Part model, mm, in its own coordinate system. Face numbers are marked on the shaded views. A direction names the side the tool comes from. Coordinates: 2 decimals unless noted, no trailing zeros. Write each loop counter-clockwise with the first axis right and the second up, starting at its lowest first coordinate (ties: lowest second). Pieces come first, ordered by that corner, then holes. Notation, with made-up numbers: M -28.75,-1.75 L -3.75,-1.75 A13 cw -3.75,20.25 Z; hole C -34,-27 d4. An arc over 180 degrees is marked long. Use a Markdown table: item, result. Add a question column.
Q1. Slice it at B-B on x = 14.5. Write the cut outline in (y, z).
Q2. Slice it at C-C on y = 9. Write the cut outline in (x, z).
Q3. Tool access for the marked faces 1, 2 and 3: list every direction of +Z, -Z, +X, -X, +Y, -Y with a clear straight run to the whole face (end or side of a thin tool).
Q4. Mould opens along Y. For the marked faces 4, 5, 6 and 7 say: released by +Y, released by -Y, zero draft, split by the parting line, or undercut.
Q5. Slice it at D-D on x = 3. Write the cut outline in (y, z), then the cut area to 3 significant figures.
Q6. Pin check, flat tips, straight feed: pin 1 Ø1.5 at (y, z) = (9.5, 1) entering from +X; pin 2 Ø4 at (x, y) = (-9.5, -10) entering from +Z; pin 3 Ø6.5 at (y, z) = (-4, -4) entering from +X. Stop position of each tip, or through.
Q7. Wall check: L1, parallel to Y at x = 2, z = 0.25; L2, parallel to Y at x = -5, z = 3; L3, parallel to X at y = 1, z = -2.5. Give the ranges that are in metal, low to high. Write a range as from..to.
Q8. Slice it at A-A on z = 1.25. Write the cut outline in (x, y).
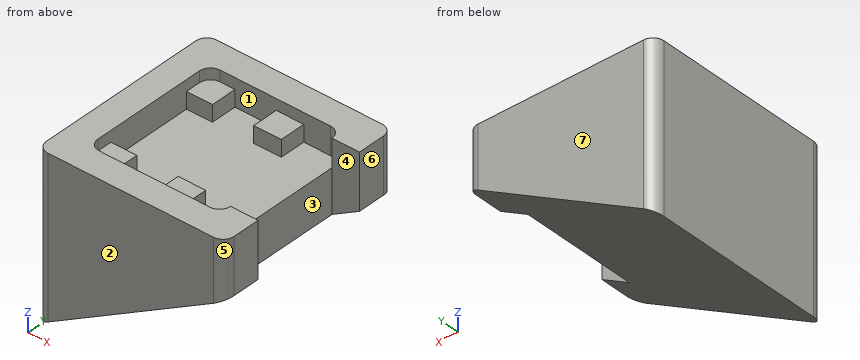
from build123d import *

# Parameters (mm, degrees)
F0_W     = 5
F0_H     = 4.7
F1_DEPTH = 5
F2_DEPTH = 3
F4_DEPTH = 2
F6_DEPTH = 35.2
F7_DEPTH = 25
F8_DEPTH = 25


with BuildPart() as f1:
    # F0 (on Top) → F1 (new body)
    with BuildSketch(Plane.XY):
        with BuildLine():
            ThreePointArc((12.031, -10.6), (11.4452135624, -12.0142135624), (10.031, -12.6))
            Line((10.031, -12.6), (5.169, -12.6))
            Line((5.169, -12.6), (0.169, -12.6))
            Line((0.169, -12.6), (-7.331, -12.6))
            Line((-7.331, -12.6), (-10.031, -12.6))
            ThreePointArc((-10.031, -12.6), (-11.4452135624, -12.0142135624), (-12.031, -10.6))
            Line((-12.031, -10.6), (-12.031, -7.9))
            Line((-12.031, -7.9), (-12.031, 7.9))
            Line((-12.031, 7.9), (-12.031, 10.6))
            ThreePointArc((-12.031, 10.6), (-11.4452135624, 12.0142135624), (-10.031, 12.6))
            Line((-10.031, 12.6), (-7.331, 12.6))
            Line((-7.331, 12.6), (0.169, 12.6))
            Line((0.169, 12.6), (5.169, 12.6))
            Line((5.169, 12.6), (10.031, 12.6))
            ThreePointArc((10.031, 12.6), (11.4452135624, 12.0142135624), (12.031, 10.6))
            Line((12.031, 10.6), (17.031, 10.6))
            Line((17.031, 10.6), (17.031, 15.6))
            ThreePointArc((17.031, 15.6), (16.4452135624, 17.0142135624), (15.031, 17.6))
            Line((15.031, 17.6), (-15.031, 17.6))
            ThreePointArc((-15.031, 17.6), (-16.4452135624, 17.0142135624), (-17.031, 15.6))
            Line((-17.031, 15.6), (-17.031, -15.6))
            ThreePointArc((-17.031, -15.6), (-16.4452135624, -17.0142135624), (-15.031, -17.6))
            Line((-15.031, -17.6), (15.031, -17.6))
            ThreePointArc((15.031, -17.6), (16.4452135624, -17.0142135624), (17.031, -15.6))
            Line((17.031, -15.6), (17.031, -10.6))
            Line((17.031, -10.6), (12.031, -10.6))
        make_face()
        with BuildLine():
            Line((5.169, -12.6), (10.031, -12.6))
            ThreePointArc((10.031, -12.6), (11.4452135624, -12.0142135624), (12.031, -10.6))
            Line((12.031, -10.6), (12.031, -10.4))
            Line((12.031, -10.4), (12.031, 10.4))
            Line((12.031, 10.4), (12.031, 10.6))
            ThreePointArc((12.031, 10.6), (11.4452135624, 12.0142135624), (10.031, 12.6))
            Line((10.031, 12.6), (5.169, 12.6))
            Line((5.169, 12.6), (5.169, 7.9))
            Line((5.169, 7.9), (0.169, 7.9))
            Line((0.169, 7.9), (0.169, 12.6))
            Line((0.169, 12.6), (-7.331, 12.6))
            Line((-7.331, 12.6), (-7.331, 7.9))
            Line((-7.331, 7.9), (-12.031, 7.9))
            Line((-12.031, 7.9), (-12.031, -7.9))
            Line((-12.031, -7.9), (-7.331, -7.9))
            Line((-7.331, -7.9), (-7.331, -12.6))
            Line((-7.331, -12.6), (0.169, -12.6))
            Line((0.169, -12.6), (0.169, -7.9))
            Line((0.169, -7.9), (5.169, -7.9))
            Line((5.169, -7.9), (5.169, -12.6))
        make_face()
        with BuildLine():
            Line((-12.031, 10.6), (-12.031, 7.9))
            Line((-12.031, 7.9), (-7.331, 7.9))
            Line((-7.331, 7.9), (-7.331, 12.6))
            Line((-7.331, 12.6), (-10.031, 12.6))
            ThreePointArc((-10.031, 12.6), (-11.4452135624, 12.0142135624), (-12.031, 10.6))
        make_face()
        with Locations((2.669, 10.25)):
            Rectangle(F0_W, F0_H)
        with Locations((2.669, -10.25)):
            Rectangle(F0_W, F0_H)
        with BuildLine():
            Line((-10.031, -12.6), (-7.331, -12.6))
            Line((-7.331, -12.6), (-7.331, -7.9))
            Line((-7.331, -7.9), (-12.031, -7.9))
            Line((-12.031, -7.9), (-12.031, -10.6))
            ThreePointArc((-12.031, -10.6), (-11.4452135624, -12.0142135624), (-10.031, -12.6))
        make_face()
    extrude(amount=-F1_DEPTH)

    # F0 (on Top) → F2 (join)
    with BuildSketch(Plane.XY):
        with BuildLine():
            ThreePointArc((12.031, -10.6), (11.4452135624, -12.0142135624), (10.031, -12.6))
            Line((10.031, -12.6), (5.169, -12.6))
            Line((5.169, -12.6), (0.169, -12.6))
            Line((0.169, -12.6), (-7.331, -12.6))
            Line((-7.331, -12.6), (-10.031, -12.6))
            ThreePointArc((-10.031, -12.6), (-11.4452135624, -12.0142135624), (-12.031, -10.6))
            Line((-12.031, -10.6), (-12.031, -7.9))
            Line((-12.031, -7.9), (-12.031, 7.9))
            Line((-12.031, 7.9), (-12.031, 10.6))
            ThreePointArc((-12.031, 10.6), (-11.4452135624, 12.0142135624), (-10.031, 12.6))
            Line((-10.031, 12.6), (-7.331, 12.6))
            Line((-7.331, 12.6), (0.169, 12.6))
            Line((0.169, 12.6), (5.169, 12.6))
            Line((5.169, 12.6), (10.031, 12.6))
            ThreePointArc((10.031, 12.6), (11.4452135624, 12.0142135624), (12.031, 10.6))
            Line((12.031, 10.6), (17.031, 10.6))
            Line((17.031, 10.6), (17.031, 15.6))
            ThreePointArc((17.031, 15.6), (16.4452135624, 17.0142135624), (15.031, 17.6))
            Line((15.031, 17.6), (-15.031, 17.6))
            ThreePointArc((-15.031, 17.6), (-16.4452135624, 17.0142135624), (-17.031, 15.6))
            Line((-17.031, 15.6), (-17.031, -15.6))
            ThreePointArc((-17.031, -15.6), (-16.4452135624, -17.0142135624), (-15.031, -17.6))
            Line((-15.031, -17.6), (15.031, -17.6))
            ThreePointArc((15.031, -17.6), (16.4452135624, -17.0142135624), (17.031, -15.6))
            Line((17.031, -15.6), (17.031, -10.6))
            Line((17.031, -10.6), (12.031, -10.6))
        make_face()
        with BuildLine():
            Line((-12.031, 10.6), (-12.031, 7.9))
            Line((-12.031, 7.9), (-7.331, 7.9))
            Line((-7.331, 7.9), (-7.331, 12.6))
            Line((-7.331, 12.6), (-10.031, 12.6))
            ThreePointArc((-10.031, 12.6), (-11.4452135624, 12.0142135624), (-12.031, 10.6))
        make_face()
        with Locations((2.669, 10.25)):
            Rectangle(F0_W, F0_H)
        with Locations((2.669, -10.25)):
            Rectangle(F0_W, F0_H)
        with BuildLine():
            Line((-10.031, -12.6), (-7.331, -12.6))
            Line((-7.331, -12.6), (-7.331, -7.9))
            Line((-7.331, -7.9), (-12.031, -7.9))
            Line((-12.031, -7.9), (-12.031, -10.6))
            ThreePointArc((-12.031, -10.6), (-11.4452135624, -12.0142135624), (-10.031, -12.6))
        make_face()
    extrude(amount=F2_DEPTH)

    # F3 (on face) → F4 (join)
    with BuildSketch(Plane.XY.offset(3)):
        with BuildLine():
            ThreePointArc((-12.031, 10.6), (-11.4452135624, 12.0142135624), (-10.031, 12.6))
            Line((-10.031, 12.6), (-7.331, 12.6))
            Line((-7.331, 12.6), (0.169, 12.6))
            Line((0.169, 12.6), (5.169, 12.6))
            Line((5.169, 12.6), (10.031, 12.6))
            ThreePointArc((10.031, 12.6), (11.4452135624, 12.0142135624), (12.031, 10.6))
            Line((12.031, 10.6), (17.031, 10.6))
            Line((17.031, 10.6), (17.031, 15.6))
            ThreePointArc((17.031, 15.6), (16.4452135624, 17.0142135624), (15.031, 17.6))
            Line((15.031, 17.6), (-15.031, 17.6))
            ThreePointArc((-15.031, 17.6), (-16.4452135624, 17.0142135624), (-17.031, 15.6))
            Line((-17.031, 15.6), (-17.031, -15.6))
            ThreePointArc((-17.031, -15.6), (-16.4452135624, -17.0142135624), (-15.031, -17.6))
            Line((-15.031, -17.6), (15.031, -17.6))
            ThreePointArc((15.031, -17.6), (16.4452135624, -17.0142135624), (17.031, -15.6))
            Line((17.031, -15.6), (17.031, -10.6))
            Line((17.031, -10.6), (12.031, -10.6))
            ThreePointArc((12.031, -10.6), (11.4452135624, -12.0142135624), (10.031, -12.6))
            Line((10.031, -12.6), (5.169, -12.6))
            Line((5.169, -12.6), (0.169, -12.6))
            Line((0.169, -12.6), (-7.331, -12.6))
            Line((-7.331, -12.6), (-10.031, -12.6))
            ThreePointArc((-10.031, -12.6), (-11.4452135624, -12.0142135624), (-12.031, -10.6))
            Line((-12.031, -10.6), (-12.031, -7.9))
            Line((-12.031, -7.9), (-12.031, 7.9))
            Line((-12.031, 7.9), (-12.031, 10.6))
        make_face()
    extrude(amount=F4_DEPTH)

    # F5 (on face) → F6 (join, through all)
    with BuildSketch(Plane(origin=(0, 17.6, 0), x_dir=(-1, 0, 0), z_dir=(0, 1, 0))):
        Polygon((17.031, -24.6657048691), (17.031, -5), (15.031, -5), (-15.031, -5), (-17.031, -5), align=None)
    extrude(amount=-F6_DEPTH)

    # F7 (cut): faces of the model
    f7_faces = [f1.faces().sort_by_distance(p)[0] for p in [
        (-16.5842641221, -17.1532641221, -5),
        (-16.5842641221, 17.1532641221, -5),
        (16.5842641221, 17.1532641221, -5),
        (16.5842641221, -17.1532641221, -5),
    ]]
    extrude(f7_faces, amount=-F7_DEPTH, mode=Mode.SUBTRACT)

    # F8 (cut): a face of the model
    f8_faces = [f1.faces().sort_by_distance(p)[0] for p in [
        (14.531, 0, -5),
    ]]
    extrude(f8_faces, amount=-F8_DEPTH, mode=Mode.SUBTRACT)


solid = f1.part
Recorded:
| question | item | result |
|---|---|---|
| 1 | outline | M -17.6,-6.46 L -10.6,-6.46 L -10.6,5 L -17.6,5 Z; M 10.6,-6.46 L 17.6,-6.46 L 17.6,5 L 10.6,5 Z |
| 2 | outline | M -17.03,-24.67 L 12.03,-7.89 L 12.03,0 L 5.17,0 L 5.17,3 L 0.17,3 L 0.17,0 L -7.33,0 L -7.33,3 L -12.03,3 L -12.03,5 L -17.03,5 Z |
| 3 | face 1 | +Z |
| 3 | face 2 | +Z, -Z, +X, -X, -Y |
| 3 | face 3 | +Z, -Z, +X |
| 4 | face 4 | undercut |
| 4 | face 5 | released by -Y |
| 4 | face 6 | zero draft |
| 4 | face 7 | released by +Y |
| 5 | outline | M -17.6,-13.1 L 17.6,-13.1 L 17.6,5 L 12.6,5 L 12.6,3 L 7.9,3 L 7.9,0 L -7.9,0 L -7.9,3 L -12.6,3 L -12.6,5 L -17.6,5 Z |
| 5 | area | 539 mm² |
| 6 | pin 1 | x = 5.17 |
| 6 | pin 2 | z = 3 |
| 6 | pin 3 | x = 12.03 |
| 7 | L1 | -17.6..-7.9, 7.9..17.6 |
| 7 | L2 | -17.6..-12.6, 12.6..17.6 |
| 7 | L3 | -17.03..12.03 |
| 8 | outline | M -17.03,-15.6 A2 ccw -15.03,-17.6 L 15.03,-17.6 A2 ccw 17.03,-15.6 L 17.03,-10.6 L 12.03,-10.6 A2 cw 10.03,-12.6 L 5.17,-12.6 L 5.17,-7.9 L 0.17,-7.9 L 0.17,-12.6 L -7.33,-12.6 L -7.33,-7.9 L -12.03,-7.9 L -12.03,7.9 L -7.33,7.9 L -7.33,12.6 L 0.17,12.6 L 0.17,7.9 L 5.17,7.9 L 5.17,12.6 L 10.03,12.6 A2 cw 12.03,10.6 L 17.03,10.6 L 17.03,15.6 A2 ccw 15.03,17.6 L -15.03,17.6 A2 ccw -17.03,15.6 Z |
